Check sheet for the modelled part. Datum: model origin and axes. Units: mm. A direction names the side the tool comes from. Give positions to 0.01 mm unless a question says otherwise; leave off trailing zeros. Write each loop counter-clockwise with the first axis right and the second up, starting at its lowest first coordinate (ties: lowest second). Pieces come first, ordered by that corner, then holes. Notation, with made-up numbers: M -4,37.25 L 40,37.25 A13 cw 40,45.25 Z; hole C 67.25,-27 d11. An arc over 180 degrees is marked long. One line per item, written item: value. Start each with the question number.
from build123d import *

# Parameters (mm, degrees)
SKETCH_1_W      = 5
SKETCH_1_H      = 2
EXTRUDE_1_DEPTH = 2
SKETCH_2_W      = 0.5
SKETCH_2_H      = 0.5
EXTRUDE_2_DEPTH = 5
SKETCH_3_W      = 1.4
SKETCH_3_H      = 1
EXTRUDE_3_DEPTH = 3


with BuildPart() as part:
    # Эскиз1 → Бобышка-Вытянуть1 (new body)
    with BuildSketch(Plane.XY):
        with Locations((2.5, -1)):
            Rectangle(SKETCH_1_W, SKETCH_1_H)
    extrude(amount=EXTRUDE_1_DEPTH)

    # Эскиз2 → Бобышка-Вытянуть2 (add)
    with BuildSketch(Plane(origin=(0, 0, 0), x_dir=(-1, 0, 0), z_dir=(0, 0, -1))):
        with Locations((-1.25, -1)):
            Rectangle(SKETCH_2_W, SKETCH_2_H)
        with Locations((-2.5, -1)):
            Rectangle(SKETCH_2_W, SKETCH_2_H)
        with Locations((-3.75, -1)):
            Rectangle(SKETCH_2_W, SKETCH_2_H)
    extrude(amount=EXTRUDE_2_DEPTH)

    # Эскиз3 → Бобышка-Вытянуть3 (add)
    with BuildSketch(Plane.XY.offset(2)):
        with Locations((2.5, -1)):
            Rectangle(SKETCH_3_W, SKETCH_3_H)
    extrude(amount=EXTRUDE_3_DEPTH)


solid = part.part
1) Cross-section at D-D (z = 3). Record the boundary of the cut face in (x, y).
2) Tool access check on faces 1 (the flat face through (3.2, -1, 3)), 2 (the flat face through (2, -0.5, 3)), 3 (the flat face through (1.8, -1, 3)), 4 (the flat face through (2, -1, 5)), 5 (the flat face through (2, -1.5, 3)). Record the directions out of +Z, -Z, +X, -X, +Y, -Y that give a thin tool (end or side, any length) a straight path to the whole face; none if there is none.
3) Cross-section at B-B (x = 2.35). Record the boundary of the cut face in (y, z).
4) Gauge pin test, flat ends, axial feed: pin 1 (0.8 mm diameter, centred on y = -1, z = 3.5, fed in from -X); pin 2 (2 mm diameter, centred on x = 2, z = 3.5, fed in from +Y); pin 3 (1 mm diameter, centred on y = -1.5, z = -3.5, fed in from +X). Record the tip position at first contact, or that the pin passes through.
5) Cross-section at C-C (y = -1.4). Record the boundary of the cut face in (x, z), plus the area to 3 significant figures.
6) Cross-section at A-A (z = -2.5). Record the boundary of the cut face in (x, y).
7) Material ranges on L1, parallel to X at y = -0.8, z = -3.75; L2, parallel to Z at x = 2.45, y = -0.6; L3, parallel to Z at x = 3.7, y = -0.4, recorded low to high. Write a range as from..to.
Data:
1. outline: M 1.8,-1.5 L 3.2,-1.5 L 3.2,-0.5 L 1.8,-0.5 Z
2. face 1: +Z, +X, +Y, -Y
2. face 2: +Z, +X, -X, +Y
2. face 3: +Z, -X, +Y, -Y
2. face 4: +Z, +X, -X, +Y, -Y
2. face 5: +Z, +X, -X, -Y
3. outline: M -2,0 L -1.25,0 L -1.25,-5 L -0.75,-5 L -0.75,0 L 0,0 L 0,2 L -0.5,2 L -0.5,5 L -1.5,5 L -1.5,2 L -2,2 Z
4. pin 1: stops at x = 1.8
4. pin 2: stops at y = -0.5
4. pin 3: stops at x = 4
5. outline: M 0,0 L 5,0 L 5,2 L 3.2,2 L 3.2,5 L 1.8,5 L 1.8,2 L 0,2 Z
5. area: 14.2 mm2
6. outline: M 1,-1.25 L 1.5,-1.25 L 1.5,-0.75 L 1,-0.75 Z; M 2.25,-1.25 L 2.75,-1.25 L 2.75,-0.75 L 2.25,-0.75 Z; M 3.5,-1.25 L 4,-1.25 L 4,-0.75 L 3.5,-0.75 Z
7. L1: x = 1..1.5, 2.25..2.75, 3.5..4
7. L2: z = 0..5
7. L3: z = 0..2
